Design review of the part built by this model. Coordinates are the model's own, in mm. Coordinates: 2 decimals unless noted, no trailing zeros. Write each loop counter-clockwise with the first axis right and the second up, starting at its lowest first coordinate (ties: lowest second). Pieces come first, ordered by that corner, then holes. Notation, with made-up numbers: (-23, 17) -> (21, 17) arc R23 ccw to (21, 47) -> close; hole circle Ø2 at (34, -2.75). An arc over 180 degrees is marked (long way). Answer in a Markdown table with one row per item. Add a question column.
Item 1: Take a section at C-C, the plane z = -83.5. Write out the cut boundary in (x, y), and give its area (4 significant figures).
Item 2: Take a section at A-A, the plane y = -3.75. Write out the cut boundary in (x, z).
Item 3: Take a section at B-B, the plane x = -48.5. Write out the cut boundary in (y, z).
Item 4: To check wall thickness, follow line 1 (X direction, y = -13.75, z = -52.5); line 2 (Z direction, x = 25, y = -12.5); line 3 (Z direction, x = 144.5, y = -17.5). State the ranges of each line that lie inside material, in increasing order.
from build123d import *

# Parameters (mm, degrees)
F0_W     = 510
F0_H     = 460
F1_DEPTH = 25
F2_W     = 325
F2_H     = 350
F3_DEPTH = 25
F4_R     = 50


with BuildPart() as f1:
    # F0 (on Front) → F1 (new body)
    with BuildSketch(Plane.XZ):
        Rectangle(F0_W, F0_H)
    extrude(amount=F1_DEPTH)

    # F2 (on face) → F3 (cut)
    with BuildSketch(Plane.XZ.offset(25)):
        with Locations((0, -10)):
            Rectangle(F2_W, F2_H)
    extrude(amount=-F3_DEPTH, mode=Mode.SUBTRACT)

    # F4
    f4_edges = [f1.edges().sort_by_distance(p)[0] for p in [
        (-162.5, -12.5, 165),
        (162.5, -12.5, 165),
        (-162.5, -12.5, -185),
        (162.5, -12.5, -185),
    ]]
    fillet(f4_edges, radius=F4_R)


solid = f1.part
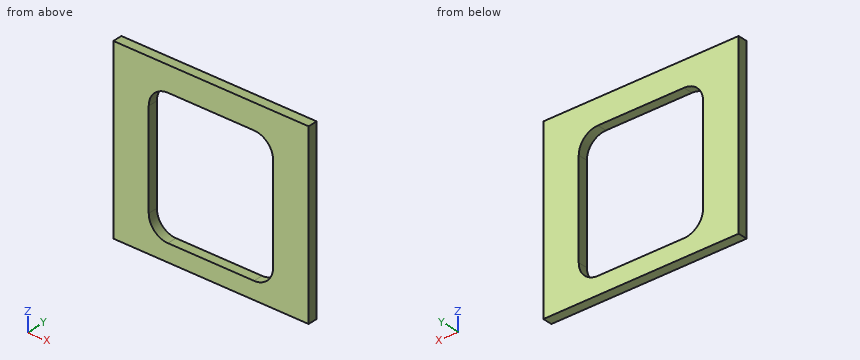
Answers:
| question | item | result |
|---|---|---|
| 1 | outline | (-255, -25) -> (-162.5, -25) -> (-162.5, 0) -> (-255, 0) -> close; (162.5, -25) -> (255, -25) -> (255, 0) -> (162.5, 0) -> close |
| 1 | area | 4,625 mm^2 |
| 2 | outline | (-255, -230) -> (255, -230) -> (255, 230) -> (-255, 230) -> close; hole (-162.5, -135) arc R50 ccw to (-112.5, -185) -> (112.5, -185) arc R50 ccw to (162.5, -135) -> (162.5, 115) arc R50 ccw to (112.5, 165) -> (-112.5, 165) arc R50 ccw to (-162.5, 115) -> close |
| 3 | outline | (-25, -230) -> (0, -230) -> (0, -185) -> (-25, -185) -> close; (-25, 165) -> (0, 165) -> (0, 230) -> (-25, 230) -> close |
| 4 | line 1 | x = -255 to -162.5, 162.5 to 255 |
| 4 | line 2 | z = -230 to -185, 165 to 230 |
| 4 | line 3 | z = -230 to -173.42, 153.42 to 230 |
